Design review of the part built by this model. Coordinates are the model's own, in mm. Round coordinates to 2 decimals unless told otherwise and drop trailing zeros. Loops run counter-clockwise (first coordinate to the right, second up) from the corner with the lowest first, then second, coordinate; pieces in that order, holes last. Notation, with made-up numbers: (-33.5, -8) - (-23.5, -8) arc R21 cw to (-23.5, -1) - close; hole circle Ø5 at (-38.5, 49.5). An arc over 180 degrees is marked (long way). Use one line per item in the form item = value. Start each with the question number.
(1) We need section B-B, the plane x = -27.5. Write out the cut boundary in (y, z), then the cut area to 3 significant figures.
(2) We need section A-A, the plane z = 4.25. Write out the cut boundary in (x, y), then the cut area to 3 significant figures.
(3) Wall thickness on probe 1 along Y at (x, z) = (2, 5.25); probe 2 along Y at (x, z) = (138, 6.5): over which ranges is each line inside the solid? List them lowest first. Write a range as [from, to].
(4) For pin 1 (1.9 mm diameter, centred on x = 98, z = 11, fed in from -Y); pin 2 (5.5 mm diameter, centred on x = 102.5, z = 7, fed in from -Y); pin 3 (3.5 mm diameter, centred on y = 6, z = 5, fed in from -X); pin 4 (1.5 mm diameter, centred on x = 69.5, y = 5, fed in from +Z), all flat-tipped, find the tip position at first contact; note any pin that passes through.
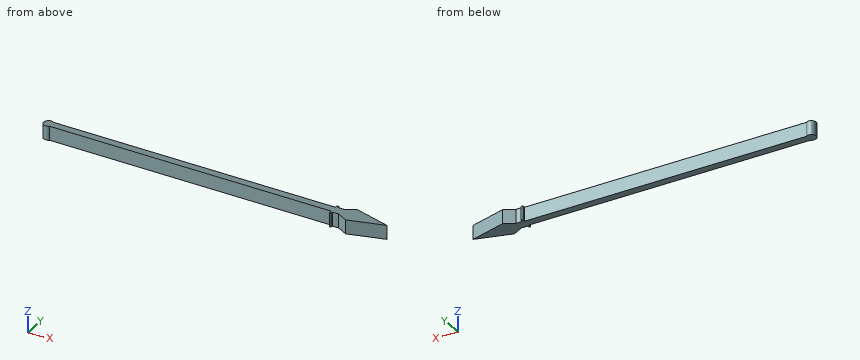
from build123d import *

# Parameters (mm, degrees)
PAD_DEPTH = 15


with BuildPart() as part:
    # Sketch001 → Pad (new body)
    with BuildSketch(Plane.XY):
        with BuildLine():
            Line((-203.120468, -3.876596), (96.879532, -3.876596))
            Line((96.879532, -7.091605), (96.879532, -3.876596))
            Line((96.879532, -7.091605), (98.646553, -7.091605))
            Line((98.646553, -7.091605), (98.646553, -4.864568))
            Line((98.646553, -4.864568), (105.327652, -4.864568))
            Line((105.327652, -4.864568), (116.029373, -10.627858))
            Line((116.029373, -10.627858), (153.887405, 0))
            Line((116.029373, 10.627858), (153.887405, 0))
            Line((105.327652, 4.864568), (116.029373, 10.627858))
            Line((98.646553, 4.864568), (105.327652, 4.864568))
            Line((98.646553, 7.091605), (98.646553, 4.864568))
            Line((96.609558, 7.091605), (98.646553, 7.091605))
            Line((96.609558, 7.091605), (96.609558, 4.065819))
            Line((-203.356306, 4.065819), (96.609558, 4.065819))
            ThreePointArc((-203.356306, 4.065819), (-211.516091, -0.151182), (-203.120468, -3.876596))
        make_face()
    extrude(amount=PAD_DEPTH)


solid = part.part
Data:
q1.outline = (-3.88, 0) - (4.07, 0) - (4.07, 15) - (-3.88, 15) - close
q1.area = 119 mm^2
q2.outline = (-203.36, 4.07) arc R5.09 ccw (long way) to (-203.12, -3.88) - (96.88, -3.88) - (96.88, -7.09) - (98.65, -7.09) - (98.65, -4.86) - (105.33, -4.86) - (116.03, -10.63) - (153.89, 0) - (116.03, 10.63) - (105.33, 4.86) - (98.65, 4.86) - (98.65, 7.09) - (96.61, 7.09) - (96.61, 4.07) - close
q2.area = 3,110 mm^2
q3.probe_1 = [-3.88, 4.07]
q3.probe_2 = [-4.46, 4.46]
q4.pin_1 = -7.09
q4.pin_2 = -4.86
q4.pin_3 = -209.23
q4.pin_4 = through
